Geometry check sheet. Reference: the model listing, model coordinates, mm. A direction names the side the tool comes from. Round coordinates to 2 decimals unless told otherwise and drop trailing zeros. Order: outer loops, then holes, each group sorted by start corner. A loop starts at its lowest first (then second) coordinate and runs counter-clockwise, first axis right, second up. Notation, with made-up numbers: (42, 65) -> (50, 65) arc R22 ccw to (50, 91) -> close; hole circle Ø2 at (51.25, 0.25). An arc over 180 degrees is marked (long way). Use a Markdown table: item, result. Add a question column.
Item 1: Mould release check, pull along Y, two halves, no side actions. Record for faces 3 (the flat face through (10, 31, 77)), 4 (the cylindrical face through (39.96, -1.81, 39.44)), 5 (the flat face through (38, 0, 0)): pulls with the +Y half, pulls with the -Y half, needs draft (parallel to the pull), parting line crosses it, or undercut.
Item 2: Sectioned sample at B-B, the plane x = 6. Record the cut outline in (y, z).
Item 3: Gauge pin test, flat ends, axial feed: pin 1 Ø6 at (x, z) = (29.5, 36.5) entering from -Y; pin 2 Ø3 at (x, y) = (12, -30) entering from -Z; pin 3 Ø6 at (y, z) = (-20, 48) entering from -X. Record the tip position at first contact, or that the pin passes through.
Item 4: Sectioned sample at A-A, the plane x = 36. Record the cut outline in (y, z), and give its area (3 significant figures).
Item 5: Sectioned sample at D-D, the plane y = 0. Record the cut outline in (x, z), and give its area (3 significant figures).
Item 6: Material ranges on probe 1 along Z at (x, y) = (21, 29); probe 2 along Y at (x, z) = (16.5, 49.5); probe 3 along Y at (x, z) = (33, 25.5), recorded low to high. Write a range as [from, to].
Item 7: Set-up check for faces 1 (the flat face through (9, -31, 77)), 2 (the cylindrical face through (7.96, 33.9, 78.48)): record each of +Z, -Z, +X, -X, +Y, -Y from which the full face is reachable in a straight line by a thin tool's end or side.
Item 8: Sectioned sample at C-C, the plane z = 58.5. Record the cut outline in (x, y).
from build123d import *

# Parameters (mm, degrees)
BOSS_EXTRUDE1_DEPTH      = 80
BOSS_EXTRUDE2_REACH      = 99.98
BOSS_EXTRUDE2_END_RADIUS = 37
SKETCH4_W                = 3
SKETCH4_H                = 10
BOSS_EXTRUDE3_REACH      = 99.98
BOSS_EXTRUDE3_END_RADIUS = 37
SKETCH5_W                = 3
SKETCH5_H                = 10
SKETCH6_R                = 3
CUT_EXTRUDE1_DEPTH       = 3


with BuildPart() as part:
    # Sketch2 → Boss-Extrude1 (new body)
    with BuildSketch(Plane.XY):
        with BuildLine():
            Line((0.933575247, 39.989103982), (0.863557104, 36.989921183))
            ThreePointArc((0.863557104, 36.989921183), (36.989921183, -0.863557104), (-0.863557104, -36.989921183))
            Line((-0.863557104, -36.989921183), (-0.933575248, -39.989103982))
            ThreePointArc((-0.933575248, -39.989103982), (39.989103982, -0.933575247), (0.933575247, 39.989103982))
        make_face()
    extrude(amount=BOSS_EXTRUDE1_DEPTH)

    # Boss-Extrude2: up to this cylinder (the profile starts inside it)
    boss_extrude2_end = Plane(origin=(0, 0, 78.5), z_dir=(0, 0, -1)) * Cylinder(BOSS_EXTRUDE2_END_RADIUS, 274.96, mode=Mode.PRIVATE)
    # Sketch4 → Boss-Extrude2 (add, up to the surface)
    with BuildSketch(Plane(origin=(0, 0, 0), x_dir=(0, 0, 1), z_dir=(-0.9997275995418874, 0.02333938118750909, 0)), mode=Mode.PRIVATE) as boss_extrude2_sk1:
        with Locations((78.5, -32)):
            Rectangle(SKETCH4_W, SKETCH4_H)
    boss_extrude2_tool1 = extrude(boss_extrude2_sk1.sketch, amount=-BOSS_EXTRUDE2_REACH, mode=Mode.PRIVATE) & boss_extrude2_end
    add(boss_extrude2_tool1.solids().sort_by_distance((-0.74686, -31.991283, 78.5))[0])

    # Boss-Extrude3: up to this cylinder (the profile starts inside it)
    boss_extrude3_end = Plane(origin=(0, 0, 78.5), z_dir=(0, 0, -1)) * Cylinder(BOSS_EXTRUDE3_END_RADIUS, 274.96, mode=Mode.PRIVATE)
    # Sketch5 → Boss-Extrude3 (add, up to the surface)
    with BuildSketch(Plane(origin=(0, 0, 0), x_dir=(0, 0, 1), z_dir=(-0.9997275995418874, 0.02333938118750974, 0)), mode=Mode.PRIVATE) as boss_extrude3_sk1:
        with Locations((78.5, 32)):
            Rectangle(SKETCH5_W, SKETCH5_H)
    boss_extrude3_tool1 = extrude(boss_extrude3_sk1.sketch, amount=-BOSS_EXTRUDE3_REACH, mode=Mode.PRIVATE) & boss_extrude3_end
    add(boss_extrude3_tool1.solids().sort_by_distance((0.74686, 31.991283, 78.5))[0])

    # Sketch6 → Cut-Extrude1 (cut)
    with BuildSketch(Plane(origin=(0, 0, 77), x_dir=(-1, 0, 0), z_dir=(0, 0, -1))):
        with Locations((-5.745498196, 31.874586279)):
            Circle(SKETCH6_R)
        with Locations((-4.2517778, -32.107980091)):
            Circle(SKETCH6_R)
    extrude(amount=-CUT_EXTRUDE1_DEPTH, mode=Mode.SUBTRACT)


solid = part.part
Found:
| question | item | result |
|---|---|---|
| 1 | face 3 | undercut |
| 1 | face 4 | parting line crosses it |
| 1 | face 5 | needs draft |
| 2 | outline | (-39.55, 0) -> (-36.51, 0) -> (-36.51, 77) -> (-34.55, 77) -> (-34.55, 80) -> (-39.55, 80) -> close; (-29.67, 77) -> (-27.15, 77) -> (-27.15, 80) -> (-29.67, 80) -> close; (26.87, 77) -> (28.89, 77) -> (28.89, 80) -> (26.87, 80) -> close; (34.86, 77) -> (36.51, 77) -> (36.51, 0) -> (39.55, 0) -> (39.55, 80) -> (34.86, 80) -> close |
| 3 | pin 1 | stops at y = -29.96 |
| 3 | pin 2 | stops at z = 77 |
| 3 | pin 3 | stops at x = 28.98 |
| 4 | outline | (-17.44, 0) -> (-8.54, 0) -> (-8.54, 80) -> (-17.44, 80) -> close; (8.54, 0) -> (17.44, 0) -> (17.44, 80) -> (8.54, 80) -> close |
| 4 | area | 1,420 mm2 |
| 5 | outline | (37, 0) -> (40, 0) -> (40, 80) -> (37, 80) -> close |
| 5 | area | 240 mm2 |
| 6 | probe 1 | z = [77, 80] |
| 6 | probe 2 | y = [-36.44, -33.12], [33.12, 36.44] |
| 6 | probe 3 | y = [-22.61, -16.73], [16.73, 22.61] |
| 7 | face 1 | -Z, -X |
| 7 | face 2 | +Z, -Z |
| 8 | outline | (-0.93, -39.99) arc R40 ccw to (0.93, 39.99) -> (0.86, 36.99) arc R37 cw to (-0.86, -36.99) -> close |
